Check sheet for the modelled part. Datum: model origin and axes. Units: mm. A direction names the side the tool comes from. Round coordinates to 2 decimals unless told otherwise and drop trailing zeros. Order: outer loops, then holes, each group sorted by start corner. A loop starts at its lowest first (then second) coordinate and runs counter-clockwise, first axis right, second up.
```python
from build123d import *

# Parameters (mm, degrees)
F1_DEPTH = 25.4
F3_DEPTH = 6.35
F5_DEPTH = 25.401
F7_DEPTH = 6.35


with BuildPart() as f1:
    # F0 (on Front) → F1 (new body)
    with BuildSketch(Plane.XZ):
        Polygon((21.227144, 31.75), (0, 31.75), (0, 0), (37.555713, 0), align=None)
        Polygon((34.47143, 31.75), (21.227144, 31.75), (37.555713, 0), (50.8, 0), align=None)
        Polygon((50.8, 31.75), (34.47143, 31.75), (50.8, 0), align=None)
    extrude(amount=-F1_DEPTH)

    # F2 (on Front) → F3 (cut, symmetric)
    with BuildSketch(Plane.XZ):
        Polygon((13.543111, 0), (28.911175, 32.08084), (0, 32.08084), (0, 0), align=None)
    extrude(amount=F3_DEPTH, both=True, mode=Mode.SUBTRACT)

    # F4 (on face) → F5 (cut, through all)
    with BuildSketch(Plane(origin=(0, 25.4, 0), x_dir=(-1, 0, 0), z_dir=(0, 1, 0))):
        Polygon((0, 31.75), (-19.05, 31.75), (0, 0), align=None)
    extrude(amount=-F5_DEPTH, mode=Mode.SUBTRACT)

    # F6 (on face) → F7 (cut, symmetric)
    with BuildSketch(Plane(origin=(0, 25.4, 0), x_dir=(-1, 0, 0), z_dir=(0, 1, 0))):
        Polygon((-19.05, 31.75), (-28.334875, 31.75), (-9.284875, 0), (0, 0), align=None)
    extrude(amount=F7_DEPTH, both=True, mode=Mode.SUBTRACT)


solid = f1.part
```
Item 1: Sectioned sample at B-B (x = 26). Record the cut outline in (y, z).
Answer:
outline: (0, 0) - (25.4, 0) - (25.4, 27.86) - (19.05, 27.86) - (19.05, 31.75) - (6.35, 31.75) - (6.35, 26) - (0, 26) - close
Item 2: Sectioned sample at D-D (x = 4.5). Record the cut outline in (y, z), and give its area (4 significant figures).
Answer:
outline: (6.35, 0) - (19.05, 0) - (19.05, 7.5) - (6.35, 7.5) - close
area: 95.25 mm2
Item 3: Access from +Z, -Z, +X, -X, +Y, -Y to the whole of each face (thin tool, end or side, straight path). Record for faces 1 (the flat face through (39, 13, 31.75)), 2 (the flat face through (14, 6.35, 16)), 3 (the flat face through (18.943, 22.269, 16.097)).
Answer:
face 1: +Z, +X, -X, +Y, -Y
face 2: +Z, -X, -Y
face 3: +Z, -X, +Y
Item 4: Sectioned sample at C-C (y = 23.25). Record the cut outline in (x, z), and give its area (3 significant figures).
Answer:
outline: (9.28, 0) - (50.8, 0) - (50.8, 31.75) - (28.33, 31.75) - close
area: 1,020 mm2
Item 5: Scan lines: line 1 along Y through (x, z) = (12, 12.5); line 2 along Y through (x, z) = (17.5, 9); line 3 along Z through (x, y) = (14, 21.75). Record each from-to range of solid material in increasing order.
Answer:
line 1: y = 6.35 to 19.05
line 2: y = 6.35 to 25.4
line 3: z = 0 to 7.86
Item 6: Go/stop test with flat-tipped pins: P1, Ø3, axis at y = 3.5, z = 4, coming from the -X side; P2, Ø1, axis at x = 43, y = 3, coming from the -Z side; P3, Ø14, axis at x = 11, z = 18, coming from the +Y side; P4, Ø2, axis at x = 15, z = 22.5, coming from the -Y side. Record where each tip stops, or that it passes through.
Answer:
P1: stops at x = 14.74
P2: stops at z = 0
P3: stops at y = 19.05
P4: stops at y = 6.35
Item 7: Sectioned sample at A-A (z = 24.5). Record the cut outline in (x, y), and give its area (3 significant figures).
Answer:
outline: (14.7, 6.35) - (25.28, 6.35) - (25.28, 0) - (50.8, 0) - (50.8, 25.4) - (23.98, 25.4) - (23.98, 19.05) - (14.7, 19.05) - close
area: 791 mm2
